```python
from build123d import *

# Parameters (mm, degrees)
BOSS_EXTRUDE1_DEPTH = 20
SKETCH3_R           = 5
CUT_EXTRUDE1_DEPTH  = 30
CUT_EXTRUDE2_START  = -30
SKETCH4_R           = 5
CUT_EXTRUDE2_DEPTH  = 30


with BuildPart() as part:
    # Sketch1 → Boss-Extrude1 (new body)
    with BuildSketch(Plane.XY):
        Polygon((-250, 240), (250, 240), (250, 120), (265, 120), (265, -240), (-265, -240), (-265, 120), (-250, 120), align=None)
    extrude(amount=BOSS_EXTRUDE1_DEPTH)

    # Sketch3 → Cut-Extrude1 (cut)
    with BuildSketch(Plane(origin=(265, 0, 0), x_dir=(0, 0, -1), z_dir=(1, 0, 0))):
        with Locations(Location((-10, -210, 0), (0, 0, 90))):
            Circle(SKETCH3_R)
        with Locations(Location((-10, -110, 0), (0, 0, 90))):
            Circle(SKETCH3_R)
        with Locations(Location((-10, -10, 0), (0, 0, 90))):
            Circle(SKETCH3_R)
        with Locations(Location((-10, 90, 0), (0, 0, 90))):
            Circle(SKETCH3_R)
    extrude(amount=-CUT_EXTRUDE1_DEPTH, mode=Mode.SUBTRACT)

    # Sketch4 → Cut-Extrude2 (cut)
    with BuildSketch(Plane.ZY.offset(265).offset(CUT_EXTRUDE2_START)):
        with Locations(Location((10, -210, 0), (0, 0, 90))):
            Circle(SKETCH4_R)
        with Locations(Location((10, -110, 0), (0, 0, 90))):
            Circle(SKETCH4_R)
        with Locations(Location((10, -10, 0), (0, 0, 90))):
            Circle(SKETCH4_R)
        with Locations(Location((10, 90, 0), (0, 0, 90))):
            Circle(SKETCH4_R)
    extrude(amount=CUT_EXTRUDE2_DEPTH, mode=Mode.SUBTRACT)


solid = part.part
```
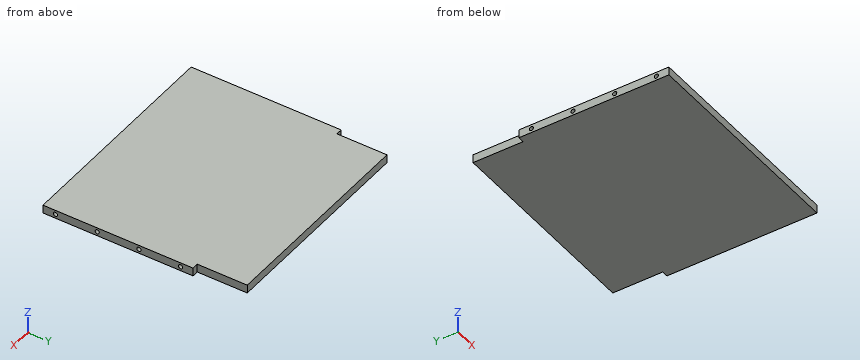
Geometry: final body of the model. Coordinates: model frame, mm. Round coordinates to 2 decimals unless told otherwise and drop trailing zeros. Loops run counter-clockwise (first coordinate to the right, second up) from the corner with the lowest first, then second, coordinate; pieces in that order, holes last. Notation, with made-up numbers: (43, 25.5) -> (75, 25.5) arc R24 ccw to (75, 39.5) -> close; hole circle Ø3 at (-26.5, 71). An arc over 180 degrees is marked (long way). Use one line per item in the form item = value.
Item 1: Contact query for flat-ended pins moving along their axis: pin 1 Ø8 at (y, z) = (-10, 10) entering from +X; pin 2 Ø6 at (y, z) = (-110, 10) entering from -X; pin 3 Ø10 at (y, z) = (179, 12.5) entering from +X. Output: stop coordinate, or through.
Evaluation:
pin_1 = 235
pin_2 = -235
pin_3 = 250
Item 2: Material intervals for probe 1 along Z at (x, y) = (255, -110); probe 2 along X at (y, z) = (200, 3.25), sorted ascending.
Evaluation:
probe_1 = 0 to 5, 15 to 20
probe_2 = -250 to 250
Item 3: Cut plane A-A on y = 189.5. Output: boundary loops of the cut face in (x, z), then the cut area to 3 significant figures.
Evaluation:
outline = (-250, 0) -> (250, 0) -> (250, 20) -> (-250, 20) -> close
area = 10,000 mm2
